Verification items for the finished model (mm, model axes). Face numbers are marked on the shaded views. A direction names the side the tool comes from. Give positions to 0.01 mm unless a question says otherwise; leave off trailing zeros. Write each loop counter-clockwise with the first axis right and the second up, starting at its lowest first coordinate (ties: lowest second). Pieces come first, ordered by that corner, then holes. Notation, with made-up numbers: (13, 5) -> (36, 5) arc R16 ccw to (36, 24) -> close; hole circle Ø3 at (28, 53.5). An arc over 180 degrees is marked (long way). Answer as CSV lines item,"result". Start each with the question number.
1) Material ranges on L1, parallel to Z at x = -24.5, y = 21.5; L2, parallel to X at y = 3.45, z = 0; L3, parallel to Y at x = 26.5, z = -26, recorded low to high.
2) Gauge pin test, flat ends, axial feed: pin 1 Ø2 at (y, z) = (33, 39) entering from +X; pin 2 Ø1 at (x, y) = (59, 55) entering from -Z; pin 3 Ø1.6 at (y, z) = (41.5, -59) entering from -X; pin 4 Ø22.5 at (y, z) = (36.5, 5) entering from +X. Record the tip position at first contact, or that the pin passes through.
3) Sectioned sample at D-D on y = 19.5. Record the cut outline in (x, z), and give its area (3 significant figures).
4) Tool access check on the marked faces 1, 2, 3 and 4. Record the directions out of +Z, -Z, +X, -X, +Y, -Y that give a thin tool (end or side, any length) a straight path to the whole face; none if there is none.
5) Sectioned sample at C-C on x = 0. Record the cut outline in (y, z).
6) Mould release check, pull along Z, two halves, no side actions. Record for the marked faces 5, 6 and 7: released by +Z, released by -Z, zero draft, split by the parting line, or undercut.
7) Sectioned sample at B-B on z = 0. Record the cut outline in (x, y), and give its area (3 significant figures).
8) Sectioned sample at A-A on y = 75.5. Record the cut outline in (x, z), and give its area (3 significant figures).
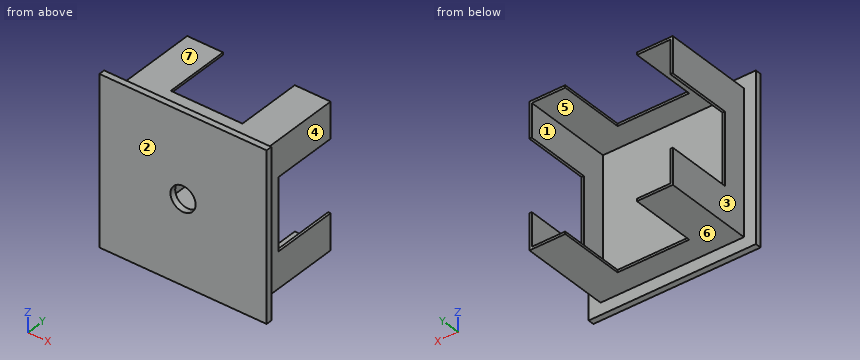
```python
from build123d import *

# Parameters (mm, degrees)
SKETCH1_W               = 140
SKETCH1_H               = 140
SKETCH1_R               = 10.5
BOSS_EXTRUDE1_DEPTH     = 5
SKETCH2_W               = 120
SKETCH2_H               = 120
SKETCH2_W_2             = 116
SKETCH2_H_2             = 116
BOSS_EXTRUDE2_DEPTH     = 75.5
CUT_EXTRUDE1_DEPTH      = 128.594082935
CUT_EXTRUDE1_DEPTH_BACK = 128.594082935
SKETCH4_W               = 60
SKETCH4_H               = 55.5
CUT_EXTRUDE2_DEPTH      = 128.594082935
CUT_EXTRUDE2_DEPTH_BACK = 128.594082935
SKETCH6_W               = 60
SKETCH6_H               = 55.5


with BuildPart() as part:
    # Sketch1 → Boss-Extrude1 (new body)
    with BuildSketch(Plane(origin=(0, 0, 0), x_dir=(1, 0, 0), z_dir=(0, 1, 0))):
        Rectangle(SKETCH1_W, SKETCH1_H)
        with Locations(Location((0, 0, 0), (0, 0, 270))):
            Circle(SKETCH1_R, mode=Mode.SUBTRACT)
    extrude(amount=BOSS_EXTRUDE1_DEPTH)

    # Sketch2 → Boss-Extrude2 (add)
    with BuildSketch(Plane(origin=(0, 5, 0), x_dir=(1, 0, 0), z_dir=(0, 1, 0))):
        Rectangle(SKETCH2_W, SKETCH2_H)
        Rectangle(SKETCH2_W_2, SKETCH2_H_2, mode=Mode.SUBTRACT)
    extrude(amount=BOSS_EXTRUDE2_DEPTH)

    # Sketch4 → Cut-Extrude1 (cut, two sides: drawn at the far end of the back side and taken through both)
    with BuildSketch(Plane(origin=(0, 0, 0), x_dir=(-1, 0, 0), z_dir=(0, 0, -1)).offset(-CUT_EXTRUDE1_DEPTH_BACK)):
        with Locations((0, 52.75)):
            Rectangle(SKETCH4_W, SKETCH4_H)
    extrude(amount=CUT_EXTRUDE1_DEPTH + CUT_EXTRUDE1_DEPTH_BACK, mode=Mode.SUBTRACT)

    # Sketch6 → Cut-Extrude2 (cut, two sides: drawn at the far end of the back side and taken through both)
    with BuildSketch(Plane(origin=(0, 0, 0), x_dir=(0, 0, -1), z_dir=(1, 0, 0)).offset(-CUT_EXTRUDE2_DEPTH_BACK)):
        with Locations((0, 52.75)):
            Rectangle(SKETCH6_W, SKETCH6_H)
    extrude(amount=CUT_EXTRUDE2_DEPTH + CUT_EXTRUDE2_DEPTH_BACK, mode=Mode.SUBTRACT)


solid = part.part
```
Ans:
1,L1,"z = -60 to -58, 58 to 60"
1,L2,"x = -70 to -10.5, 10.5 to 70"
1,L3,"y = 0 to 5"
2,pin 1,"stops at x = 60"
2,pin 2,"stops at z = -60"
2,pin 3,"stops at x = -60"
2,pin 4,"passes through"
3,outline,"(-60, -60) -> (60, -60) -> (60, 60) -> (-60, 60) -> close; hole (-58, -58) -> (58, -58) -> (58, 58) -> (-58, 58) -> close"
3,area,"944 mm²"
4,face 1,"+Y"
4,face 2,"+Z, -Z, +X, -X, -Y"
4,face 3,"+Z, -Z, -X, +Y"
4,face 4,"+Z, -Z, +X, +Y"
5,outline,"(0, -70) -> (5, -70) -> (5, -60) -> (25, -60) -> (25, -58) -> (5, -58) -> (5, -10.5) -> (0, -10.5) -> close; (0, 10.5) -> (5, 10.5) -> (5, 58) -> (25, 58) -> (25, 60) -> (5, 60) -> (5, 70) -> (0, 70) -> close"
6,face 5,"undercut"
6,face 6,"released by -Z"
6,face 7,"released by +Z"
7,outline,"(-70, 0) -> (-10.5, 0) -> (-10.5, 5) -> (-58, 5) -> (-58, 25) -> (-60, 25) -> (-60, 5) -> (-70, 5) -> close; (10.5, 0) -> (70, 0) -> (70, 5) -> (60, 5) -> (60, 25) -> (58, 25) -> (58, 5) -> (10.5, 5) -> close"
7,area,"675 mm²"
8,outline,"(-60, -60) -> (-30, -60) -> (-30, -58) -> (-58, -58) -> (-58, -30) -> (-60, -30) -> close; (-60, 30) -> (-58, 30) -> (-58, 58) -> (-30, 58) -> (-30, 60) -> (-60, 60) -> close; (30, -60) -> (60, -60) -> (60, -30) -> (58, -30) -> (58, -58) -> (30, -58) -> close; (30, 58) -> (58, 58) -> (58, 30) -> (60, 30) -> (60, 60) -> (30, 60) -> close"
8,area,"464 mm²"
